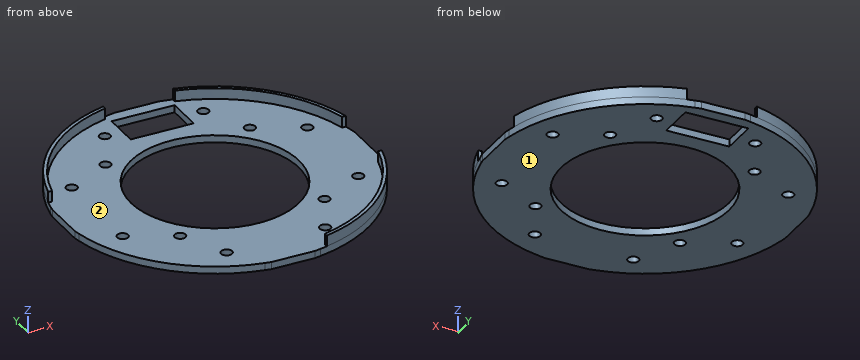
from build123d import *

# Parameters (mm, degrees)
EXTRUDE_1_DEPTH          = 2
HOLE_WIZARD_3_0_3_1_D    = 3
HOLE_WIZARD_M421_D       = 46
FILLET_1_R               = 42
EXTRUDE_2_DEPTH          = 3
PATTERN_CIRCULAR_1_COUNT = 3
PATTERN_CIRCULAR_1_ANGLE = 180
SKETCH_12_W              = 17.29
SKETCH_12_H              = 10.1
CUT_EXTRUDE_2_DEPTH      = 10


with BuildPart() as part:
    # Эскиз1 → Бобышка-Вытянуть1 (new body)
    with BuildSketch(Plane.XY.offset(-2)):
        Polygon((41.5, 6), (35.95120701, 35.95120701), (6, 41.5), (-6, 41.5), (-35.95120701, 35.95120701), (-41.5, 6), (-41.5, -6), (-35.95120701, -35.95120701), (-6, -41.5), (6, -41.5), (35.95120701, -35.95120701), (41.5, -6), align=None)
    extrude(amount=-EXTRUDE_1_DEPTH)

    # Диаметр отверстия Ø3.0 (3)1 (through all)
    with Locations(Plane.XY.offset(-2)):
        with Locations((32.291639785, -13.5), (32.291639785, 13.5), (19.798989873, 19.798989873), (19.798989873, -19.798989873), (13.5, -32.291639785), (-13.5, -32.291639785), (-19.798989873, -19.798989873), (-19.798989873, 19.798989873), (-13.5, 32.291639785), (13.5, 32.291639785), (-32.291639785, 13.5), (-32.291639785, -13.5)):
            Hole(HOLE_WIZARD_3_0_3_1_D / 2)

    # Отверстие с зазором M421 (through all)
    with Locations(Plane.XY.offset(-2)):
        with Locations((0, 0)):
            Hole(HOLE_WIZARD_M421_D / 2)

    # Скругление1
    fillet_1_edges = [part.edges().sort_by_distance(p)[0] for p in [
        (35.95120701, -35.95120701, -3),
        (-35.95120701, -35.95120701, -3),
        (-35.95120701, 35.95120701, -3),
        (35.95120701, 35.95120701, -3),
    ]]
    fillet(fillet_1_edges, radius=FILLET_1_R)

    # Эскиз10 → Бобышка-Вытянуть2 (add)
    with BuildSketch(Plane.XY.offset(-2)):
        with BuildLine():
            Line((-9.549876115, 39.769458963), (-9.549876115, 40.792474564))
            ThreePointArc((-9.549876115, 40.792474564), (-29.611492945, 29.611492945), (-40.792474564, 9.549876115))
            Line((-40.792474564, 9.549876115), (-39.769458963, 9.549876115))
            ThreePointArc((-39.769458963, 9.549876115), (-28.920667351, 28.920667351), (-9.549876115, 39.769458963))
        make_face()
    extrude_2 = extrude(amount=EXTRUDE_2_DEPTH)

    # Круговой массив1: Бобышка-Вытянуть2 ×3 about axis
    pattern_circular_1_axis = Axis((0, 0, 0), (0, 0, -1))
    for i in range(1, PATTERN_CIRCULAR_1_COUNT):
        add(extrude_2.rotate(pattern_circular_1_axis, i * PATTERN_CIRCULAR_1_ANGLE / (PATTERN_CIRCULAR_1_COUNT - 1)))

    # Эскиз12 → Вырез-Вытянуть2 (cut)
    with BuildSketch(Plane(origin=(0, 0, -4), x_dir=(-1, 0, 0), z_dir=(0, 0, -1))):
        with Locations((0, 33.05)):
            Rectangle(SKETCH_12_W, SKETCH_12_H)
    extrude(amount=-CUT_EXTRUDE_2_DEPTH, mode=Mode.SUBTRACT)


solid = part.part
Can you work these out from the model? Positions are in its coordinate system, mm. Face numbers are marked on the shaded views. Coordinates: 2 decimals unless noted, no trailing zeros. Order: outer loops, then holes, each group sorted by start corner. A loop starts at its lowest first (then second) coordinate and runs counter-clockwise, first axis right, second up. Notation, with made-up numbers: (87.25, 63.5) - (142.25, 63.5) arc R25 cw to (142.25, 78.5) - close; hole circle Ø3 at (-12.5, 83). An arc over 180 degrees is marked (long way). Answer as a JSON object with one key per item and string values. Group by question number.
Q1. Imagine slicing it at C-C (x = -13.5). Please give me the cut outline in (y, z).
Q2. Imagine slicing it at D-D (y = 13.5). Please give me the cut outline in (x, z).
Q3. Will these pins go through, and if not, where does the flat tip stop? P1, Ø1.8, axis at x = -32.29, y = -13.5, coming from the +Z side; P2, Ø3.5, axis at x = 32.29, y = -13.5, coming from the +Z side; P3, Ø0.5, axis at x = -40, z = -1, coming from the -Y side; P4, Ø1, axis at y = -13.5, z = -3, coming from the +X side.
Q4. Imagine slicing it at A-A (x = 0). Please give me the cut outline in (y, z).
Q5. We'd pull the mould along Y, two halves only. Please class the marked faces 1 and 2: +Y half, -Y half, draft (parallel to the pull), parting line (faces both ways), or undercut.
Q6. Imagine slicing it at B-B (y = 0). Please give me the cut outline in (x, z), and give its area (3 significant figures).
Q7. I need wall thicknesses on line 1 (Y direction, x = -3, z = -2.3); line 2 (Y direction, x = 8, z = -2.9); line 3 (X direction, y = -14, z = -2.65). Which ranges of each line are inside material? Lowest first, please. Write a range as from..to.
Determined:
{
 "1": {"outline": "(-39.65, -4) - (-33.79, -4) - (-33.79, -2) - (-39.65, -2) - close; (-30.79, -4) - (-18.62, -4) - (-18.62, -2) - (-30.79, -2) - close; (18.62, -4) - (30.79, -4) - (30.79, -2) - (18.62, -2) - close; (33.79, -4) - (39.65, -4) - (39.65, 1) - (38.61, 1) - (38.61, -2) - (33.79, -2) - close"},
 "2": {"outline": "(-39.65, -4) - (-33.79, -4) - (-33.79, -2) - (-38.61, -2) - (-38.61, 1) - (-39.65, 1) - close; (-30.79, -4) - (-18.62, -4) - (-18.62, -2) - (-30.79, -2) - close; (18.62, -4) - (30.79, -4) - (30.79, -2) - (18.62, -2) - close; (33.79, -4) - (39.65, -4) - (39.65, 1) - (38.61, 1) - (38.61, -2) - (33.79, -2) - close"},
 "3": {"P1": "passes through", "P2": "stops at z = -2", "P3": "stops at y = 9.55", "P4": "stops at x = 39.82"},
 "4": {"outline": "(-41.5, -4) - (-23, -4) - (-23, -2) - (-41.5, -2) - close; (23, -4) - (28, -4) - (28, -2) - (23, -2) - close; (38.1, -4) - (41.5, -4) - (41.5, -2) - (38.1, -2) - close"},
 "5": {"face 1": "draft", "face 2": "undercut"},
 "6": {"outline": "(-41.5, -4) - (-23, -4) - (-23, -2) - (-41.5, -2) - close; (23, -4) - (41.5, -4) - (41.5, -2) - (23, -2) - close", "area": "74.0 mm2"},
 "7": {"line 1": "y = -41.5..-22.8, 22.8..28, 38.1..41.5", "line 2": "y = -41.13..-21.56, 21.56..28, 38.1..41.13", "line 3": "x = -39.48..-33.71, -30.88..-18.25, 18.25..30.88, 33.71..39.48"}
}
